Autodesk Inventor part; units mm, degrees
ref_plane "YZ Plane" through (0, 0, 0) normal (1, 0, 0) x (0, 1, 0)
ref_plane "XZ Plane" through (0, 0, 0) normal (0, 1, 0) x (-1, 0, 0)
ref_plane "XY Plane" through (0, 0, 0) normal (0, 0, 1) x (1, 0, 0)
sketch "スケッチ1" plane through (0, 0, 0) normal (0, 0, 1) x (1, 0, 0)
  line L0 (0, 0) -> (6, 0) construction
  line L1 (0, -3.25) -> (6, -3.25)
  line L2 (6, 3.25) -> (0, 3.25)
  arc A0 (0, 3.25) -> (0, -3.25) centre (0, 0) ccw
  arc A1 (6, -3.25) -> (6, 3.25) centre (6, 0) ccw
  line L3 (-15, 0) -> (-9, 0) construction
  line L4 (-9, 3.25) -> (-15, 3.25)
  arc A2 (-15, 3.25) -> (-18.25, 0) centre (-15, 0) ccw
  arc A3 (-9, -3.25) -> (-9, 3.25) centre (-9, 0) ccw
  line L5 (-9, 0) -> (0, 0)
  circle A4 centre (-15, 0) radius 3.25 construction
  circle A5 centre (2.6047, -14.7721) radius 3.25
  line L6 (0, 0) -> (2.6047, -14.7721) construction
  arc A6 (-11.2916, -3.25) -> (2.0404, -11.5715) centre (0, 0) ccw
  line L7 (0, 0) -> (125.4, 0)
  line L8 (125.262, -9.9907) -> (5.461, -13.2216)
  line L9 (-11.2916, -3.25) -> (-9, -3.25)
  arc A7 (-11.75, 0) -> (-11.2916, -3.25) centre (0, 0) ccw
  arc A8 (2.0404, -11.5715) -> (-11.75, 0) centre (0, 0) ccw
  line L10 (9.9117, 6.3104) -> (125.4, 0)
  line L11 (-9.9117, 6.3104) -> (9.9117, 6.3104)
  line L12 (-15, 6.3104) -> (-15, 0) construction
  circle A9 centre (125.1272, -4.9926) radius 5
  line L13 (8.7592, -7.832) -> (125.262, -9.9907)
  circle A10 centre (-11.8389, 5.95) radius 1.5
  arc A11 (-13.6588, 2.9604) -> (-8.835, 7.7463) centre (-11.8389, 5.95) ccw
  arc A12 (-8.835, 7.7463) -> (-10.9368, 9.3317) centre (-11.8389, 5.95) ccw construction
  arc A13 (-14.066, 3.25) -> (-13.6588, 2.9604) centre (-11.8389, 5.95) ccw
  line L14 (-11.8389, 5.95) -> (-10.9368, 9.3317)
  arc A14 (-10.9368, 9.3317) -> (-14.066, 3.25) centre (-11.8389, 5.95) ccw
  point P0 (3, 0)
  point P1 (-12, 0)
  point P2 (2.0404, -11.5715)
  point P3 (124.8544, 0)
  point P4 (11.75, 0)
  point P5 (124.8073, -9.9823)
  point P6 (-11.2916, 3.25)
  point P7 (-10.4987, 5.2764)
  point P8 (-11.4523, 7.3993)
  point P9 (-11.488, 2.4676)
  dimension "d7" = 6.5
  dimension "d0" = 6.5
  dimension "d1" = 6
  dimension "d3" = 6.5
  dimension "d4" = 6
  dimension "d5" = 15
  dimension "d6" = 6.5
  dimension "d8" = 15
  dimension "d9" = 100
  dimension "d11" = 125.4
  dimension "d18" = 10
  dimension "d26" = 3
  dimension "d27" = 2
  dimension "d28" = 1.2
extrude "押し出し1" add sketch "スケッチ1" along normal blind 5 contours L1 A1 L7 A8 A6 L9 A3 L5 A0 | L5 A3 L4 A11 L11 A8 L7 A1 L2 A0 | A8 L10 A9 L7 | A9 L7 | L7 A9 L13 A8 | A9 L7 | L4 A8 L11 A11 | L4 A14 L14 A10 A8
fillet "フィレット2" radius 2 1 edges at (8.7592, -7.832, 2.5)
properties part number "Wing2" material "ポリカーボネート、クリア"
Can you work these out from the model? Positions are in its coordinate system, mm. A direction names the side the tool comes from. Give positions to 0.01 mm unless a question says otherwise; leave off trailing zeros. Loops run counter-clockwise (first coordinate to the right, second up) from the corner with the lowest first, then second, coordinate; pieces in that order, holes last. Notation, with made-up numbers: M -23.5,1.25 L 15.5,1.25 A24 ccw 15.5,29.25 Z; hole C 52.5,60.25 d1. An arc over 180 degrees is marked long. One line per item, written item: value. Start each with the question number.
1) If we section it at A-A, the plane z = 3.6: Write out the boundary of the cut face in (x, y), and give its area (3 significant figures).
2) If I drill on line 1 (Y direction, x = 5, z = 4.7); line 2 (Y direction, x = 9.5, z = 2.55); line 3 (Y direction, x = -7, z = 1.1), over which ranges is the centre line in solid material (lowest first)? Write a range as [from, to].
3) If we section it at C-C, the plane x = 78.5: Write out the boundary of the cut face in (y, z).
4) I'm going to push flat-ended pins straight in: pin 1 (2.5 mm diameter, centred on x = 4, z = 2.5, fed in from +Y); pin 2 (1.5 mm diameter, centred on y = -1, z = 2.5, fed in from +X); pin 3 (6 mm diameter, centred on x = 105.5, y = 4.5, fed in from -Z); pin 4 (2.5 mm diameter, centred on x = -11.5, z = 2.5, fed in from -Y). Where does each tip first touch, or does it pass through?
5) If we section it at B-B, the plane x = 24: Write out the boundary of the cut face in (y, z), and give its area (3 significant figures).
6) On a 3-axis mill with a long thin cutter (end or side, diameter ignored), from which of +Z, -Z, +X, -X, +Y, -Y can I reach the whole of each face in a straight line? I mean faces 1 (the face through (-10, -3.25, 2)), 2 (the face through (0, 6.31, 2)), 3 (the face through (9.25, 0.07, 2.46)), 4 (the face through (130.127, -4.955, 2.465)), 5 (the face through (56, -3, 0)). Say none if no direction works.
7) Thinking about a two-plate mould opening in Y: for faces 6 (the face through (66.8, 3.2, 2.5)), 7 (the face through (-5.75, 0.07, 2.46)), 8 (the face through (56, -3, 5)), which applies, +Y half, -Y half, draft (parallel to the pull), parting line (faces both ways), or undercut?
Completed:
1. outline: M -14.07,3.25 L -9,3.25 A3.25 cw -9,-3.25 L -11.29,-3.25 A11.75 ccw 2.04,-11.57 A11.75 ccw 8.2,-8.42 A2 cw 9.63,-7.85 L 125.26,-9.99 A5 ccw 125.4,0 L 9.91,6.31 L -9.91,6.31 A11.75 ccw -10.5,5.28 A1.5 cw long -11.45,7.4 L -10.94,9.33 A3.5 ccw Z; hole M 0,-3.25 L 6,-3.25 A3.25 ccw 6,3.25 L 0,3.25 A3.25 ccw Z
1. area: 1,690 mm^2
2. line 1: y = [-10.63, -3.25], [3.25, 6.31]
2. line 2: y = [-7.85, 6.31]
2. line 3: y = [-9.44, -2.56], [2.56, 6.31]
3. outline: M -9.12,0 L 2.56,0 L 2.56,5 L -9.12,5 Z
4. pin 1: stops at y = 6.31
4. pin 2: stops at x = 128.93
4. pin 3: passes through
4. pin 4: stops at y = -5.74
5. outline: M -8.11,0 L 5.54,0 L 5.54,5 L -8.11,5 Z
5. area: 68.3 mm^2
6. face 1: +Z, -Z, -X
6. face 2: +Z, -Z, +X, +Y
6. face 3: +Z, -Z
6. face 4: +Z, -Z, +X
6. face 5: -Z, +X, -X, +Y, -Y
7. face 6: +Y half
7. face 7: undercut
7. face 8: draft
